```python
from build123d import *

# Parameters (mm, degrees)
F1_DEPTH     = 3.81
F2_R         = 0.762
F3_R         = 0.508
F4_R         = 0.381
F5_T1_DEPTH  = 0.6101247647
F5_T3_DEPTH  = 3.3655
F5_T5_DEPTH  = 5.8289214894
F5_T7_DEPTH  = 0.4831247647
F5_T9_DEPTH  = 5.8289214894
F5_T11_DEPTH = 3.048
F5_S15_W     = 0.381
F5_S15_H     = 0.381
F5_T16_DEPTH = 0.381
F5_S21_W     = 0.381
F5_S21_H     = 0.381
F5_T22_DEPTH = 0.381
F5_S27_W     = 0.381
F5_S27_H     = 0.381
F5_T28_DEPTH = 0.381
F5_S33_W     = 0.381
F5_S33_H     = 0.381
F5_T34_DEPTH = 0.381
F5_T38_ANGLE = 90
F5_T40_ANGLE = 67.60378922
F5_T42_ANGLE = 135.20757844
F5_T44_ANGLE = 67.60378922
F5_T46_ANGLE = 233.4571121673
F5_T48_ANGLE = 90
F7_DEPTH     = 2.54


# Not quite as in the source:
# - a fillet or chamfer that OpenCascade refuses, or shapes differently, is made with other operations: its cross-section is extruded or revolved along the edge and cut away or added


with BuildPart() as f1:
    # F0 (on Top) → F1 (new body)
    with BuildSketch(Plane.XY):
        with BuildLine():
            Line((0, -4.2545), (0, -8.509))
            Line((0, -8.509), (5.2574214894, -8.509))
            ThreePointArc((5.2574214894, -8.509), (7.3025, -6.4639214894), (9.3475785106, -8.509))
            Line((9.3475785106, -8.509), (14.605, -8.509))
            Line((14.605, -8.509), (14.605, -4.2545))
            Line((14.605, -4.2545), (13.081, -4.2545))
            ThreePointArc((13.081, -4.2545), (7.366, -0.0716128896), (1.651, -4.2545))
            Line((1.651, -4.2545), (0, -4.2545))
        make_face()
    extrude(amount=F1_DEPTH)

    # F2
    f2_edges = [f1.edges().sort_by_distance(p)[0] for p in [
        (13.081, -4.2545, 1.905),
        (1.651, -4.2545, 1.905),
    ]]
    fillet(f2_edges, radius=F2_R)

    # F3
    f3_edges = [f1.edges().sort_by_distance(p)[0] for p in [
        (0, -4.2545, 1.905),
        (14.605, -4.2545, 1.905),
    ]]
    fillet(f3_edges, radius=F3_R)

    # F4
    f4_edges = [f1.edges().sort_by_distance(p)[0] for p in [
        (0.813062, -4.2545, 0),
        (0.14879, -4.40329, 0),
        (1.542043, -4.125696, 0),
        (0, -6.63575, 0),
        (7.366, -0.071613, 0),
        (2.628711, -8.509, 0),
        (13.189957, -4.125696, 0),
        (7.3025, -6.463921, 0),
        (13.855438, -4.2545, 0),
        (11.976289, -8.509, 0),
        (14.45621, -4.40329, 0),
        (14.605, -6.63575, 0),
    ]]
    fillet(f4_edges, radius=F4_R)

    # F5: fillet of radius 0.381 on 14 edges, made by hand

    # F5_s2 → F5_t1 (cut)
    with BuildSketch(Plane.YZ.offset(0.508)):
        with BuildLine():
            ThreePointArc((-4.2545, 3.429), (-4.3660923164, 3.6984076836), (-4.6355, 3.81))
            Line((-4.6355, 3.81), (-4.2545, 3.81))
            Line((-4.2545, 3.81), (-4.2545, 3.429))
        make_face()
    extrude(amount=F5_T1_DEPTH, mode=Mode.SUBTRACT)

    # F5_s4 → F5_t3 (cut)
    with BuildSketch(Plane.XZ.offset(4.7625)):
        with BuildLine():
            ThreePointArc((0.381, 3.81), (0.1115923164, 3.6984076836), (0, 3.429))
            Line((0, 3.429), (0, 3.81))
            Line((0, 3.81), (0.381, 3.81))
        make_face()
        with BuildLine():
            ThreePointArc((14.224, 3.81), (14.4934076836, 3.6984076836), (14.605, 3.429))
            Line((14.605, 3.429), (14.605, 3.81))
            Line((14.605, 3.81), (14.224, 3.81))
        make_face()
    extrude(amount=F5_T3_DEPTH, mode=Mode.SUBTRACT)

    # F5_s6 → F5_t5 (cut)
    with BuildSketch(Plane.YZ.offset(0.381)):
        with BuildLine():
            ThreePointArc((-8.128, 3.81), (-8.3974076836, 3.6984076836), (-8.509, 3.429))
            Line((-8.509, 3.429), (-8.509, 3.81))
            Line((-8.509, 3.81), (-8.128, 3.81))
        make_face()
    extrude(amount=F5_T5_DEPTH, mode=Mode.SUBTRACT)

    # F5_s8 → F5_t7 (cut)
    with BuildSketch(Plane.YZ.offset(13.6138752353)):
        with BuildLine():
            ThreePointArc((-4.6355, 3.81), (-4.3660923164, 3.6984076836), (-4.2545, 3.429))
            Line((-4.2545, 3.429), (-4.2545, 3.81))
            Line((-4.2545, 3.81), (-4.6355, 3.81))
        make_face()
    extrude(amount=F5_T7_DEPTH, mode=Mode.SUBTRACT)

    # F5_s10 → F5_t9 (cut)
    with BuildSketch(Plane.YZ.offset(8.3950785106)):
        with BuildLine():
            ThreePointArc((-8.128, 3.81), (-8.3974076836, 3.6984076836), (-8.509, 3.429))
            Line((-8.509, 3.429), (-8.509, 3.81))
            Line((-8.509, 3.81), (-8.128, 3.81))
        make_face()
    extrude(amount=F5_T9_DEPTH, mode=Mode.SUBTRACT)

    # F5_s12 → F5_t11 (cut)
    with BuildSketch(Plane.XY.offset(0.381)):
        with BuildLine():
            ThreePointArc((0, -8.128), (0.1115923164, -8.3974076836), (0.381, -8.509))
            Line((0.381, -8.509), (0, -8.509))
            Line((0, -8.509), (0, -8.128))
        make_face()
        with BuildLine():
            ThreePointArc((14.224, -8.509), (14.4934076836, -8.3974076836), (14.605, -8.128))
            Line((14.605, -8.128), (14.605, -8.509))
            Line((14.605, -8.509), (14.224, -8.509))
        make_face()
    extrude(amount=F5_T11_DEPTH, mode=Mode.SUBTRACT)


with BuildPart() as f5_tool14:
    # F5_s15 → F5_t16 (new body)
    with BuildSketch(Plane.XZ.offset(8.128)):
        with Locations((14.4145, 0.1905)):
            Rectangle(F5_S15_W, F5_S15_H)
    extrude(amount=F5_T16_DEPTH)

    # F5_s17 → F5_t18 (revolve, cut)
    with BuildSketch(Plane(origin=(14.224, -8.128, 0.381), x_dir=(-0.7071067812, 0, 0.7071067812), z_dir=(0.7071067812, 0, 0.7071067812))):
        with BuildLine():
            ThreePointArc((0, -0.381), (0.381, 0), (0, 0.381))
            Line((0, 0.381), (0, -0.381))
        make_face()
    revolve(axis=Axis((14.224, -8.128, 0.381), (0, -1, 0)), mode=Mode.SUBTRACT)


with BuildPart() as f1_1:
    add(f1.part)

    # F5_t13: cut F5_tool14
    add(f5_tool14.part, mode=Mode.SUBTRACT)


with BuildPart() as f5_tool20:
    # F5_s21 → F5_t22 (new body)
    with BuildSketch(Plane.YZ.offset(0.381)):
        with Locations((-8.3185, 0.1905)):
            Rectangle(F5_S21_W, F5_S21_H)
    extrude(amount=-F5_T22_DEPTH)

    # F5_s23 → F5_t24 (revolve, cut)
    with BuildSketch(Plane(origin=(0.381, -8.128, 0.381), x_dir=(0, 0.7071067812, 0.7071067812), z_dir=(0, -0.7071067812, 0.7071067812))):
        with BuildLine():
            ThreePointArc((0, -0.381), (0.381, 0), (0, 0.381))
            Line((0, 0.381), (0, -0.381))
        make_face()
    revolve(axis=Axis((0.381, -8.128, 0.381), (-1, 0, 0)), mode=Mode.SUBTRACT)


with BuildPart() as f1_2:
    add(f1_1.part)

    # F5_t19: cut F5_tool20
    add(f5_tool20.part, mode=Mode.SUBTRACT)


with BuildPart() as f5_tool26:
    # F5_s27 → F5_t28 (new body)
    with BuildSketch(Plane.XZ.offset(8.128)):
        with Locations((0.1905, 3.6195)):
            Rectangle(F5_S27_W, F5_S27_H)
    extrude(amount=F5_T28_DEPTH)

    # F5_s29 → F5_t30 (revolve, cut)
    with BuildSketch(Plane(origin=(0.381, -8.128, 3.429), x_dir=(0.7071067812, 0, -0.7071067812), z_dir=(-0.7071067812, 0, -0.7071067812))):
        with BuildLine():
            ThreePointArc((0, -0.381), (0.381, 0), (0, 0.381))
            Line((0, 0.381), (0, -0.381))
        make_face()
    revolve(axis=Axis((0.381, -8.128, 3.429), (0, -1, 0)), mode=Mode.SUBTRACT)


with BuildPart() as f1_3:
    add(f1_2.part)

    # F5_t25: cut F5_tool26
    add(f5_tool26.part, mode=Mode.SUBTRACT)


with BuildPart() as f5_tool32:
    # F5_s33 → F5_t34 (new body)
    with BuildSketch(Plane.YZ.offset(14.224)):
        with Locations((-8.3185, 3.6195)):
            Rectangle(F5_S33_W, F5_S33_H)
    extrude(amount=F5_T34_DEPTH)

    # F5_s35 → F5_t36 (revolve, cut)
    with BuildSketch(Plane(origin=(14.224, -8.128, 3.429), x_dir=(0, 0.7071067812, -0.7071067812), z_dir=(0, -0.7071067812, -0.7071067812))):
        with BuildLine():
            ThreePointArc((0, -0.381), (0.381, 0), (0, 0.381))
            Line((0, 0.381), (0, -0.381))
        make_face()
    revolve(axis=Axis((14.224, -8.128, 3.429), (1, 0, 0)), mode=Mode.SUBTRACT)


with BuildPart() as f1_4:
    add(f1_3.part)

    # F5_t31: cut F5_tool32
    add(f5_tool32.part, mode=Mode.SUBTRACT)

    # F5_s37 → F5_t38 (revolve, cut)
    with BuildSketch(Plane.YZ.offset(0.508)):
        with BuildLine():
            ThreePointArc((-4.2545, 3.429), (-4.3660923164, 3.6984076836), (-4.6355, 3.81))
            Line((-4.6355, 3.81), (-4.2545, 3.81))
            Line((-4.2545, 3.81), (-4.2545, 3.429))
        make_face()
    revolve(axis=Axis((0.508, -4.7625, 3.81), (0, 0, 1)), revolution_arc=F5_T38_ANGLE, mode=Mode.SUBTRACT)

    # F5_s39 → F5_t40 (revolve, cut)
    with BuildSketch(Plane.YZ.offset(1.1181247647)):
        with BuildLine():
            ThreePointArc((-4.6355, 3.81), (-4.3660923164, 3.6984076836), (-4.2545, 3.429))
            Line((-4.2545, 3.429), (-4.2545, 3.81))
            Line((-4.2545, 3.81), (-4.6355, 3.81))
        make_face()
    revolve(axis=Axis((1.1181247647, -3.4925, 3.81), (0, 0, 1)), revolution_arc=F5_T40_ANGLE, mode=Mode.SUBTRACT)

    # F5_s41 → F5_t42 (revolve, cut)
    with BuildSketch(Plane(origin=(3.2066030929, -7.7812628503, 0), x_dir=(0, 0, 1), z_dir=(0.3810092313, -0.9245712334, 0))):
        with BuildLine():
            ThreePointArc((3.81, -10.113322678), (3.6984076836, -10.3827303617), (3.429, -10.494322678))
            Line((3.429, -10.494322678), (3.81, -10.494322678))
            Line((3.81, -10.494322678), (3.81, -10.113322678))
        make_face()
    revolve(axis=Axis((7.366, -6.0672049597, 3.81), (0, 0, 1)), revolution_arc=F5_T42_ANGLE, mode=Mode.SUBTRACT)

    # F5_s43 → F5_t44 (revolve, cut)
    with BuildSketch(Plane.YZ.offset(13.6138752353)):
        with BuildLine():
            ThreePointArc((-4.6355, 3.81), (-4.3660923164, 3.6984076836), (-4.2545, 3.429))
            Line((-4.2545, 3.429), (-4.2545, 3.81))
            Line((-4.2545, 3.81), (-4.6355, 3.81))
        make_face()
    revolve(axis=Axis((13.6138752353, -3.4925, 3.81), (0, 0, -1)), revolution_arc=F5_T44_ANGLE, mode=Mode.SUBTRACT)

    # F5_s45 → F5_t46 (revolve, cut)
    with BuildSketch(Plane(origin=(4.8953206605, -9.721188669, 0), x_dir=(0, 0, 1), z_dir=(0.449764197, -0.8931473378, 0))):
        with BuildLine():
            ThreePointArc((3.81, -0.2690863714), (3.6984076836, -0.5384940551), (3.429, -0.6500863714))
            Line((3.429, -0.6500863714), (3.81, -0.6500863714))
            Line((3.81, -0.6500863714), (3.81, -0.2690863714))
        make_face()
    revolve(axis=Axis((7.3025, -8.509, 3.81), (0, 0, -1)), revolution_arc=F5_T46_ANGLE, mode=Mode.SUBTRACT)

    # F5_s47 → F5_t48 (revolve, cut)
    with BuildSketch(Plane.YZ.offset(14.097)):
        with BuildLine():
            ThreePointArc((-4.6355, 3.81), (-4.3660923164, 3.6984076836), (-4.2545, 3.429))
            Line((-4.2545, 3.429), (-4.2545, 3.81))
            Line((-4.2545, 3.81), (-4.6355, 3.81))
        make_face()
    revolve(axis=Axis((14.097, -4.7625, 3.81), (0, 0, -1)), revolution_arc=F5_T48_ANGLE, mode=Mode.SUBTRACT)

    # F6 (on face) → F7 (cut)
    with BuildSketch(Plane.XY.offset(3.81)):
        Polygon((1.3930101413, -5.4594320245), (1.3930101413, -8.8049108163), (1.3930101413, -9.2631950974), (13.2167544216, -9.2631950974), (13.2167544216, -5.4594320245), (10.9711596742, -5.4594320245), (10.9711596742, -2.5722389109), (3.5011197906, -2.5722389109), (3.5011197906, -5.4594320245), align=None)
    extrude(amount=-F7_DEPTH, mode=Mode.SUBTRACT)


solid = f1_4.part
```
For this review, take the finished solid that the model builds, in its own axes (mm). A direction names the side the tool comes from. Coordinates: 2 decimals unless noted, no trailing zeros. Write each loop counter-clockwise with the first axis right and the second up, starting at its lowest first coordinate (ties: lowest second). Pieces come first, ordered by that corner, then holes. Notation, with made-up numbers: (23.5, 61) - (79.5, 61) arc R8 ccw to (79.5, 71) - close; hole circle Ø9 at (9, -24). An arc over 180 degrees is marked (long way). Put each result on its own line as item: value.
1. Machinability: for faces 5 (the flat face through (7, -2, 3.81)), 6 (the flat face through (2, -5.459, 3)), which of the approach directions +Z, -Z, +X, -X, +Y, -Y give a long, thin tool a straight path to every point of the face, cutting with its end or side? Answer none if there is none.
Values found:
face 5: +Z, +X, -X, +Y, -Y
face 6: +Z, -Y
2. For pin 1 (1.5 mm diameter, centred on x = 2, z = 2.5, fed in from +Y); pin 2 (1.5 mm diameter, centred on x = 9.5, y = -4.5, fed in from +Z); pin 3 (1.5 mm diameter, centred on x = 8, y = -5.5, fed in from -Z); pin 4 (0.7 mm diameter, centred on x = 1, z = 1, fed in from +Y), all flat-tipped, find the tip position at first contact; note any pin that passes through.
Values found:
pin 1: y = -2.24
pin 2: z = 1.27
pin 3: z = 0
pin 4: y = -4.22
3. Add section A-A, the plane z = 0.7. Give the boundary of the cut face in (x, y) (1 decimal).
Values found:
outline: (0, -8.1) arc R0.4 ccw to (0.4, -8.5) - (5.3, -8.5) arc R2 cw to (9.3, -8.5) - (14.2, -8.5) arc R0.4 ccw to (14.6, -8.1) - (14.6, -4.8) arc R0.5 ccw to (14.1, -4.3) - (13.6, -4.3) arc R0.8 cw to (12.9, -3.8) arc R6 ccw to (1.8, -3.8) arc R0.8 cw to (1.1, -4.3) - (0.5, -4.3) arc R0.5 ccw to (0, -4.8) - close
4. Mouldability with a two-part tool opening along X and no side actions: class faces 1 (the flat face through (12, -8.509, 1)), 2 (the flat face through (7, -2.572, 3)), 3 (the flat face through (14.605, -6, 2)), 4 (the flat face through (0, -6, 2)) as released by +X, released by -X, zero draft, split by the parting line, or undercut.
Values found:
face 1: zero draft
face 2: undercut
face 3: released by +X
face 4: released by -X
5. Wall thickness on probe 1 along X at (y, z) = (-6, 2.45) (3 decimals); probe 2 along X at (y, z) = (-6.75, 0.85) (3 decimals); probe 3 along Z at (x, y) = (4.5, -2.75): over which ranges is each line inside the solid? List them lowest first.
Values found:
probe 1: 0 to 1.393, 13.217 to 14.605
probe 2: 0 to 6.259, 8.346 to 14.605
probe 3: 0 to 1.27
